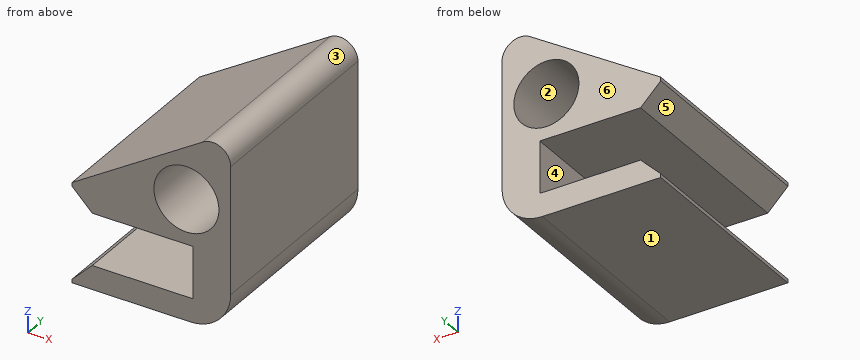
from build123d import *

# Parameters (mm, degrees)
F1_DEPTH      = 25.4
F2_DEPTH      = 25.4
F3_R          = 5.08
F4_R          = 2.286
F5_SIZE       = 2.54
F6_R          = 4.0996644409
F7_DEPTH      = 25.4
F7_DEPTH_BACK = 254


with BuildPart() as f1:
    # F0 (on Front) → F1 (new body)
    with BuildSketch(Plane.XZ):
        Polygon((-15.24, 0), (0, 0), (0, -6.55), (-15.24, -6.55), (-15.24, -9.55), (4.76, -9.55), (4.76, 3), (-15.24, 3), align=None)
    extrude(amount=F1_DEPTH)

    # F0 (on Front) → F2 (join)
    with BuildSketch(Plane.XZ):
        Polygon((4.76, 15.7), (-15.24, 3), (4.76, 3), align=None)
    extrude(amount=F2_DEPTH)

    # F3
    f3_edges = [f1.edges().sort_by_distance(p)[0] for p in [
        (4.76, -12.7, -9.55),
    ]]
    fillet(f3_edges, radius=F3_R)

    # F4
    f4_edges = [f1.edges().sort_by_distance(p)[0] for p in [
        (4.76, -12.7, 15.7),
    ]]
    fillet(f4_edges, radius=F4_R)

    # F5
    f5_edges = [f1.edges().sort_by_distance(p)[0] for p in [
        (-15.24, -12.7, 0),
        (-15.24, -12.7, -6.55),
    ]]
    chamfer(f5_edges, length=F5_SIZE)

    # F6 (on Front) → F7 (cut, two sides)
    with BuildSketch(Plane.XZ) as f7_sk:
        with Locations((-0.8245132631, 5.626801867)):
            Circle(F6_R)
    extrude(amount=-F7_DEPTH, mode=Mode.SUBTRACT)
    extrude(f7_sk.sketch, amount=F7_DEPTH_BACK, mode=Mode.SUBTRACT)


solid = f1.part
Part model, mm, in its own coordinate system. Face numbers are marked on the shaded views. A direction names the side the tool comes from. Round coordinates to 2 decimals unless told otherwise and drop trailing zeros. Write each loop counter-clockwise with the first axis right and the second up, starting at its lowest first coordinate (ties: lowest second). Pieces come first, ordered by that corner, then holes. Notation, with made-up numbers: (-23.75, -23.5) - (-6.75, -23.5) arc R16 cw to (-6.75, -3.5) - close; hole circle Ø7 at (16.5, 41). An arc over 180 degrees is marked (long way). Use CSV: the item, a comma, the result in double quotes.
Item 1: Wall check: L1, parallel to Z at x = -0.5, y = -3; L2, parallel to Z at x = -3, y = -16.75; L3, parallel to Z at x = -5.5, y = -10.75. Give the ranges that are in metal, low to high.
Results list:
L1,"z = -9.55 to -6.55, 0 to 1.54, 9.71 to 12.36"
L2,"z = -9.55 to -6.55, 0 to 2.15, 9.1 to 10.77"
L3,"z = -9.55 to -6.55, 0 to 9.18"
Item 2: Pull direction Z, two halves, no side cores. Call the marked faces 1, 2, 3 and 4: pulls with the +Z half, pulls with the -Z half, needs draft (parallel to the pull), parting line crosses it, or undercut.
Results list:
face 1,"pulls with the -Z half"
face 2,"undercut"
face 3,"pulls with the +Z half"
face 4,"undercut"
Item 3: Slice it at A-A, the plane x = -5.5. Write the cut outline in (y, z), then the cut area to 3 significant figures.
Results list:
outline,"(-25.4, -9.55) - (0, -9.55) - (0, -6.55) - (-25.4, -6.55) - close; (-25.4, 0) - (0, 0) - (0, 9.18) - (-25.4, 9.18) - close"
area,"309 mm²"
Item 4: Slice it at D-D, the plane x = -2.25. Write the cut outline in (y, z).
Results list:
outline,"(-25.4, -9.55) - (0, -9.55) - (0, -6.55) - (-25.4, -6.55) - close; (-25.4, 0) - (0, 0) - (0, 1.78) - (-25.4, 1.78) - close; (-25.4, 9.47) - (0, 9.47) - (0, 11.25) - (-25.4, 11.25) - close"
Item 5: Tool access for the marked faces 5 and 6: list every direction of +Z, -Z, +X, -X, +Y, -Y with a clear straight run to the whole face (end or side of a thin tool).
Results list:
face 5,"-X, +Y, -Y"
face 6,"+Z, -Z, +X, -X, +Y"
Item 6: Slice it at C-C, the plane y = -5. Write the cut outline in (x, z), then the cut area to 3 significant figures.
Results list:
outline,"(-15.24, -9.55) - (-0.32, -9.55) arc R5.08 ccw to (4.76, -4.47) - (4.76, 11.54) arc R2.29 ccw to (1.25, 13.47) - (-15.24, 3) - (-15.24, 2.54) - (-12.7, 0) - (0, 0) - (0, -6.55) - (-12.7, -6.55) - (-15.24, -9.09) - close; hole circle Ø8.2 at (-0.82, 5.63)"
area,"209 mm²"
Item 7: Slice it at B-B, the plane z = 9.25. Write the cut outline in (x, y).
Results list:
outline,"(-5.4, -25.4) - (-2.74, -25.4) - (-2.74, 0) - (-5.4, 0) - close; (1.09, -25.4) - (4.76, -25.4) - (4.76, 0) - (1.09, 0) - close"
Item 8: Flat gauge pins, fed straight in: P1, Ø6, axis at y = -3.5, z = 6.5, coming from the -X side; P2, Ø6.5, axis at x = -6.5, y = -13.5, coming from the +Z side; P3, Ø2, axis at y = -8, z = -3, coming from the -X side; P4, Ø4, axis at x = -12.5, z = -3.5, coming from the +Y side. Where does each tip first touch, or does it go through?
Results list:
P1,"stops at x = -14.45"
P2,"stops at z = 10.61"
P3,"stops at x = 0"
P4,"passes through"
